from build123d import *

# Parameters (mm, degrees)
SKETCH1_W           = 42
SKETCH1_H           = 35
SKETCH1_R           = 1.75
SKETCH1_R_2         = 6
SKETCH1_R_3         = 2.5
BOSS_EXTRUDE1_DEPTH = 3
SKETCH2_W           = 42
SKETCH2_H           = 3
BOSS_EXTRUDE2_DEPTH = 20
SKETCH3_R           = 3
CUT_EXTRUDE1_DEPTH  = 20
FILLET1_R           = 11


with BuildPart() as part:
    # Sketch1 → Boss-Extrude1 (new body)
    with BuildSketch(Plane(origin=(0, 0, 0), x_dir=(1, 0, 0), z_dir=(0, 1, 0))):
        with Locations((21, -17.5)):
            Rectangle(SKETCH1_W, SKETCH1_H)
        with Locations(Location((5, -10, 0), (0, 0, 270))):
            Circle(SKETCH1_R, mode=Mode.SUBTRACT)
        with Locations(Location((5, -27, 0), (0, 0, 270))):
            Circle(SKETCH1_R, mode=Mode.SUBTRACT)
        with Locations(Location((25, -18.5, 0), (0, 0, 270))):
            Circle(SKETCH1_R_2, mode=Mode.SUBTRACT)
        with Locations(Location((35, -18.5, 0), (0, 0, 270))):
            Circle(SKETCH1_R_3, mode=Mode.SUBTRACT)
    extrude(amount=BOSS_EXTRUDE1_DEPTH)

    # Sketch2 → Boss-Extrude2 (add)
    with BuildSketch(Plane.XZ):
        with Locations((21, 1.5)):
            Rectangle(SKETCH2_W, SKETCH2_H)
    extrude(amount=BOSS_EXTRUDE2_DEPTH)

    # Sketch3 → Cut-Extrude1 (cut)
    with BuildSketch(Plane(origin=(0, 0, 0), x_dir=(-1, 0, 0), z_dir=(0, 0, -1))):
        with Locations((-32, -10)):
            Circle(SKETCH3_R)
        with Locations((-10, -10)):
            Circle(SKETCH3_R)
    extrude(amount=-CUT_EXTRUDE1_DEPTH, mode=Mode.SUBTRACT)

    # Fillet1
    fillet1_edges = [part.edges().sort_by_distance(p)[0] for p in [
        (42, 1.5, 35),
        (0, 1.5, 35),
    ]]
    fillet(fillet1_edges, radius=FILLET1_R)


solid = part.part
The model under review builds one solid part; all positions refer to its coordinate system, in mm. A direction names the side the tool comes from. Coordinates: 2 decimals unless noted, no trailing zeros. Loops run counter-clockwise (first coordinate to the right, second up) from the corner with the lowest first, then second, coordinate; pieces in that order, holes last.
(1) Draft analysis for pull direction Y (two halves, no side actions). For faces 1 (the cylindrical face through (3.45, 1.48, 10.81)), 2 (the flat face through (21, -20, 2)), 3 (the cylindrical face through (35, -10, 1)), state which applies: +Y half, -Y half, draft (parallel to the pull), parting line (faces both ways), or undercut.
Determined:
face 1: draft
face 2: -Y half
face 3: undercut
(2) Consider section D-D, the plane x = 5. Give the boundary of the cut face in (y, z).
Determined:
outline: (-20, 0) - (3, 0) - (3, 8.25) - (0, 8.25) - (0, 3) - (-20, 3) - close; (0, 11.75) - (3, 11.75) - (3, 25.25) - (0, 25.25) - close; (0, 28.75) - (3, 28.75) - (3, 33.22) - (0, 33.22) - close
(3) Consider section B-B, the plane y = -9.5. Give the boundary of the cut face in (x, z), plus the area to 3 significant figures.
Determined:
outline: (0, 0) - (7.04, 0) - (7.04, 3) - (0, 3) - close; (12.96, 0) - (29.04, 0) - (29.04, 3) - (12.96, 3) - close; (34.96, 0) - (42, 0) - (42, 3) - (34.96, 3) - close
area: 90.5 mm2
(4) Tool access review of faces 4 (the flat face through (21, -10, 3)), 5 (the cylindrical face through (35, 1, 16)): name each direction out of +Z, -Z, +X, -X, +Y, -Y from which nothing blocks a thin tool from reaching the whole face with its end or side.
Determined:
face 4: +Z, +X, -X, -Y
face 5: +Y, -Y
(5) Consider section C-C, the plane x = 32. Give the boundary of the cut face in (y, z).
Determined:
outline: (-20, 0) - (-13, 0) - (-13, 3) - (-20, 3) - close; (-7, 0) - (3, 0) - (3, 34.95) - (0, 34.95) - (0, 3) - (-7, 3) - close
(6) Consider section A-A, the plane z = 10. Give the boundary of the cut face in (x, y).
Determined:
outline: (0, 0) - (3.25, 0) - (3.25, 3) - (0, 3) - close; (6.75, 0) - (42, 0) - (42, 3) - (6.75, 3) - close
(7) Insertion check: P1, Ø4, axis at x = 5, z = 10, coming from the +Y side; P2, Ø4, axis at x = 32.5, y = -14, coming from the +Z side; P3, Ø4, axis at y = 0.5, z = 26.5, coming from the -X side; P4, Ø2, axis at x = 11.5, z = 6, coming from the -Y side. Each pin has a flat end and moves straight along its axis. Give the tip position at first contact, or say it passes through.
Determined:
P1: stops at y = 3
P2: stops at z = 3
P3: stops at x = 0.01
P4: stops at y = 0
(8) Wall thickness on L1, parallel to X at y = 1.35, z = 18.5; L2, parallel to Y at x = 31, z = 7: over which ranges is each line inside the solid? List them lowest first.
Determined:
L1: x = 0 to 19, 31 to 32.5, 37.5 to 42
L2: y = 0 to 3
